Verification items for the finished model (mm, model axes). A direction names the side the tool comes from. Give positions to 0.01 mm unless a question says otherwise; leave off trailing zeros. Order: outer loops, then holes, each group sorted by start corner. A loop starts at its lowest first (then second) coordinate and runs counter-clockwise, first axis right, second up.
(1) Scan lines: L1, parallel to Y at x = 0, z = 90; L2, parallel to X at y = 1, z = 96; L3, parallel to Z at x = 7.5, y = -14.5. Record each from-to range of solid material in increasing order.
(2) Access from +Z, -Z, +X, -X, +Y, -Y to the whole of each face (thin tool, end or side, straight path). Record for faces 1 (the face through (-5.506, 24.796, 56.695)), 2 (the face through (-5.506, 24.796, -6.521)), 3 (the face through (-23.3, -14.9, 117)).
(3) Sectioned sample at C-C on z = 78. Record the cut outline in (x, y), plus the area to 3 significant figures.
(4) Sectioned sample at A-A on x = 0. Record the cut outline in (y, z).
(5) Gauge pin test, flat ends, axial feed: pin 1 (10 mm diameter, centred on x = -5, z = 50, fed in from +Y); pin 2 (1 mm diameter, centred on y = -7, z = 85, fed in from -X); pin 3 (1.5 mm diameter, centred on x = -17, y = 5.5, fed in from -Z). Record the tip position at first contact, or that the pin passes through.
(6) Mould release check, pull along Y, two halves, no side actions. Record for faces 4 (the face through (-30.37, -1.34, 54.36)), 5 (the face through (0, 0, -5)), 6 (the face through (23.3, -14.9, -10)): pulls with the +Y half, pulls with the -Y half, needs draft (parallel to the pull), parting line crosses it, or undercut.
```python
from build123d import *

# Parameters (mm, degrees)
F3_R = 2
F4_R = 2


with BuildPart() as f2:
    # F1 (on Front) → F2 (revolve)
    with BuildSketch(Plane.XZ):
        Polygon((25.4, 0), (0, 0), (0, -5), (25.4, -5), (25.4, -10), (30.4, -10), (30.4, 117), (25.4, 117), align=None)
    revolve(axis=Axis((0, 0, 13.367524), (0, 0, -1)))

    # F3
    f3_edges = [f2.edges().sort_by_distance(p)[0] for p in [
        (-30.4, 0, 117),
        (-25.4, 0, 117),
    ]]
    fillet(f3_edges, radius=F3_R)

    # F4
    f4_edges = [f2.edges().sort_by_distance(p)[0] for p in [
        (-25.4, 0, -10),
        (-30.4, 0, -10),
    ]]
    fillet(f4_edges, radius=F4_R)


solid = f2.part
```
Ans:
1. L1: y = -30.4 to -25.4, 25.4 to 30.4
1. L2: x = -30.38 to -25.38, 25.38 to 30.38
1. L3: z = -5 to 0
2. face 1: +Z
2. face 2: -Z
2. face 3: +Z, +X, -X, +Y, -Y
3. outline: circle Ø60.8 at (0, 0); hole circle Ø50.8 at (0, 0)
3. area: 877 mm2
4. outline: (-30.4, -8) arc R2 ccw to (-28.4, -10) - (-27.4, -10) arc R2 ccw to (-25.4, -8) - (-25.4, -5) - (25.4, -5) - (25.4, -8) arc R2 ccw to (27.4, -10) - (28.4, -10) arc R2 ccw to (30.4, -8) - (30.4, 115) arc R2 ccw to (28.4, 117) - (27.4, 117) arc R2 ccw to (25.4, 115) - (25.4, 0) - (-25.4, 0) - (-25.4, 115) arc R2 ccw to (-27.4, 117) - (-28.4, 117) arc R2 ccw to (-30.4, 115) - close
5. pin 1: stops at y = 30.4
5. pin 2: stops at x = -29.7
5. pin 3: stops at z = -5
6. face 4: parting line crosses it
6. face 5: undercut
6. face 6: needs draft
